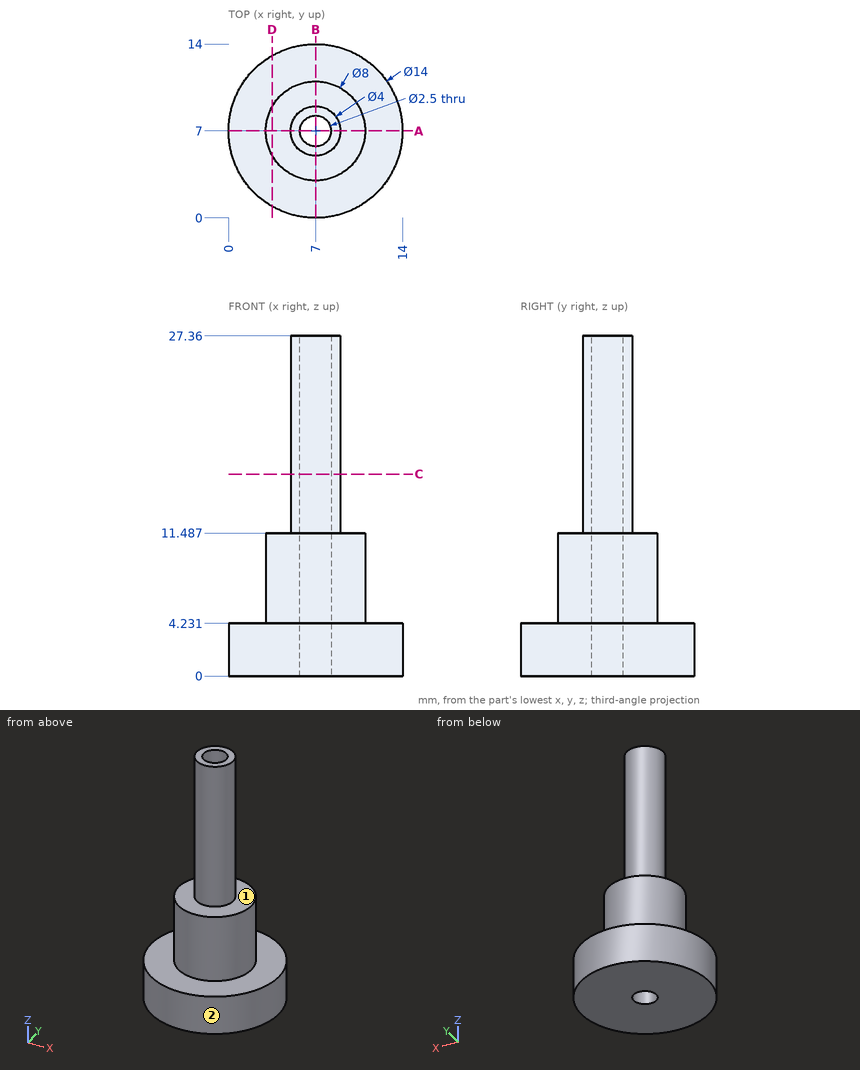
Answer from the drawing. Dimensions are ordinates in mm from the lowest x, y and z of the part. A direction names the side the tool comes from. Give positions to 0.01 mm unless a question says otherwise; leave off trailing zeros. Loops run counter-clockwise (first coordinate to the right, second up) from the corner with the lowest first, then second, coordinate; pieces in that order, holes last. Notation, with made-up numbers: (36.25, 21.5) -> (56.25, 21.5) arc R25 ccw to (56.25, 47.5) -> close; hole circle Ø5 at (35.5, 17.25). An arc over 180 degrees is marked (long way). Use a Markdown table: item, result.
Q1. Section D-D, the plane x = 3.5 is taken. Determine the outline of the cut face in (y, z).
Solved:
| item | result |
|---|---|
| outline | (0.94, 0) -> (13.06, 0) -> (13.06, 4.23) -> (8.94, 4.23) -> (8.94, 11.49) -> (5.06, 11.49) -> (5.06, 4.23) -> (0.94, 4.23) -> close |
Q2. Section C-C, the plane z = 16.25 is taken. Determine the outline of the cut face in (x, y).
Solved:
| item | result |
|---|---|
| outline | circle Ø4 at (7, 7); hole circle Ø2.5 at (7, 7) |
Q3. A tool of negligible diameter and unlimited length cuts with its end or side. For the marked faces 1 and 2, from which of +Z, -Z, +X, -X, +Y, -Y can it reach the whole face along a straight path? Write none if from no direction.
Solved:
| item | result |
|---|---|
| face 1 | +Z |
| face 2 | +Z, -Z |
Q4. Section A-A, the plane y = 7 is taken. Determine the outline of the cut face in (x, z), then the cut area to 3 significant figures.
Solved:
| item | result |
|---|---|
| outline | (0, 0) -> (5.75, 0) -> (5.75, 27.36) -> (5, 27.36) -> (5, 11.49) -> (3, 11.49) -> (3, 4.23) -> (0, 4.23) -> close; (8.25, 0) -> (14, 0) -> (14, 4.23) -> (11, 4.23) -> (11, 11.49) -> (9, 11.49) -> (9, 27.36) -> (8.25, 27.36) -> close |
| area | 112 mm^2 |
Q5. Find the intervals of material crossed by line 1 along X through (y, z) = (7, 13.5); line 2 along Y through (x, z) = (7, 9.25), in increasing order.
Solved:
| item | result |
|---|---|
| line 1 | x = 5 to 5.75, 8.25 to 9 |
| line 2 | y = 3 to 5.75, 8.25 to 11 |
Q6. Each of these flat-tipped pins is pushed along its axis until it touches: pin 1 (6.5 mm diameter, centred on x = 5.5, y = 8.5, fed in from +Z); pin 2 (6 mm diameter, centred on x = 2.5, y = 4.5, fed in from +Z); pin 3 (6 mm diameter, centred on x = 4.5, z = 12.5, fed in from +Y); pin 4 (6 mm diameter, centred on y = 12.5, z = 24, fed in from -X). Where does it stop, or does it pass through?
Solved:
| item | result |
|---|---|
| pin 1 | stops at z = 27.36 |
| pin 2 | stops at z = 11.49 |
| pin 3 | stops at y = 11 |
| pin 4 | passes through |
